```python
from build123d import *

# Parameters (mm, degrees)
F0_W        = 127
F0_H        = 88.9
F1_DEPTH    = 12.7
F2_T1_DEPTH = 177
F3_W        = 1.8
F3_H        = 6.85
F4_DEPTH    = 16.4
F3_W_2      = 7
F3_H_2      = 13.5
F3_W_3      = 2.7532497272
F3_H_3      = 12.2928316705
F5_DEPTH    = 16.4
F6_SIZE     = 1
F7_DEPTH    = 2.794
F8_DEPTH    = 1.8542
F3_R        = 3.9463270772
F9_DEPTH    = 0.762
F10_R       = 0.254
F13_W       = 127
F13_H       = 12.192
F14_DEPTH   = 0.5
F15_R       = 3.9211509086
F16_DEPTH   = 1.27


# Not quite as in the source:
# - a fillet or chamfer that OpenCascade refuses, or shapes differently, is made with other operations: its cross-section is extruded or revolved along the edge and cut away or added
# - the program builds the solid bodies; features that only make, move or delete a surface that nothing else refers to are left out


with BuildPart() as f1:
    # F0 (on Front) → F1 (new body)
    with BuildSketch(Plane.XZ):
        Rectangle(F0_W, F0_H)
    extrude(amount=F1_DEPTH)

    # F2: fillet of radius 10 on 4 edges, made by hand

    # F2_s2 → F2_t1 (cut)
    with BuildSketch(Plane.YZ.offset(-88.5)):
        with BuildLine():
            ThreePointArc((-2.7, 44.45), (-9.7710678119, 41.5210678119), (-12.7, 34.45))
            Line((-12.7, 34.45), (-12.7, 44.45))
            Line((-12.7, 44.45), (-2.7, 44.45))
        make_face()
        with BuildLine():
            ThreePointArc((-10, 44.45), (-2.9289321881, 41.5210678119), (0, 34.45))
            Line((0, 34.45), (0, 44.45))
            Line((0, 44.45), (-10, 44.45))
        make_face()
        with BuildLine():
            ThreePointArc((-2.7, -44.45), (-9.7710678119, -41.5210678119), (-12.7, -34.45))
            Line((-12.7, -34.45), (-12.7, -44.45))
            Line((-12.7, -44.45), (-2.7, -44.45))
        make_face()
        with BuildLine():
            ThreePointArc((-10, -44.45), (-2.9289321881, -41.5210678119), (0, -34.45))
            Line((0, -34.45), (0, -44.45))
            Line((0, -44.45), (-10, -44.45))
        make_face()
    extrude(amount=F2_T1_DEPTH, mode=Mode.SUBTRACT)

    # F3 (on face) → F4 (cut)
    with BuildSketch(Plane.YZ.offset(63.5)):
        with Locations((-7.1068273082, -6.4043554038)):
            Rectangle(F3_W, F3_H)
    extrude(amount=-F4_DEPTH, mode=Mode.SUBTRACT)

    # F3 (on face) → F5 (cut)
    with BuildSketch(Plane.YZ.offset(63.5)):
        with Locations((-6.591425851, 10.4809925538)):
            Rectangle(F3_W_2, F3_H_2)
        with Locations((-7.9680507146, 10.4750713799)):
            Rectangle(F3_W_3, F3_H_3, mode=Mode.SUBTRACT)
        with Locations((-6.591425851, 28.0195952505)):
            Rectangle(F3_W_2, F3_H_2)
        with Locations((-7.9680507146, 28.0764119234)):
            Rectangle(F3_W_3, F3_H_3, mode=Mode.SUBTRACT)
    extrude(amount=-F5_DEPTH, mode=Mode.SUBTRACT)

    # F6
    f6_edges = [f1.edges().sort_by_distance(p)[0] for p in [
        (55.3, -6.206827, -2.979355),
        (55.3, -6.206827, -9.829355),
    ]]
    chamfer(f6_edges, length=F6_SIZE)

    # F7 (add): faces of the model
    f7_faces = [f1.faces().sort_by_distance(p)[0] for p in [
        (63.5, -7.9680507146, 10.4750713799),
        (63.5, -7.9680507146, 28.0764119234),
    ]]
    extrude(f7_faces, amount=-F7_DEPTH)

    # F8 (cut): faces of the model
    f8_faces = [f1.faces().sort_by_distance(p)[0] for p in [
        (63.5, -7.9680507146, 10.4750713799),
        (63.5, -7.9680507146, 28.0764119234),
    ]]
    extrude(f8_faces, amount=-F8_DEPTH, mode=Mode.SUBTRACT)

    # F3 (on face) → F9 (join)
    with BuildSketch(Plane.YZ.offset(63.5)):
        with Locations((-6.3012135215, -31.0900993645)):
            Circle(F3_R)
    extrude(amount=F9_DEPTH)

    # F10
    f10_edges = [f1.edges().sort_by_distance(p)[0] for p in [
        (64.262, -10.247541, -31.090099),
    ]]
    fillet(f10_edges, radius=F10_R)

    # F13 (on face) → F14 (join)
    with BuildSketch(Plane.XZ.offset(12.7)):
        with Locations((0, 27.0355174699)):
            Rectangle(F13_W, F13_H)
        with Locations((-2.0266e-06, 13.3711864791)):
            Rectangle(F13_W, F13_H)
        with Locations((-2.0266e-06, -0.2175037199)):
            Rectangle(F13_W, F13_H)
        with Locations((-2.0266e-06, -13.8689222195)):
            Rectangle(F13_W, F13_H)
        with Locations((-2.0266e-06, -27.337996141)):
            Rectangle(F13_W, F13_H)
    extrude(amount=F14_DEPTH)

    # F15 (on face) → F16 (cut)
    with BuildSketch(Plane(origin=(-63.5, 0, 0), x_dir=(0, -1, 0), z_dir=(-1, 0, 0))):
        with Locations((7.0751463063, -30.106594786)):
            Circle(F15_R)
        with Locations((7.0751463063, 29.6837498702)):
            Circle(F15_R)
    extrude(amount=-F16_DEPTH, mode=Mode.SUBTRACT)

    # F17: fillet of radius 2.54 on 2 edges, made by hand

    # F17_s1 → F17_t2 (revolve)
    with BuildSketch(Plane.XY.offset(-30.106594786)):
        with BuildLine():
            ThreePointArc((-63.5, -10.9962972149), (-62.5702954744, -10.0665926893), (-62.23, -8.7965926893))
            Line((-62.23, -8.7965926893), (-62.23, -10.9962972149))
            Line((-62.23, -10.9962972149), (-63.5, -10.9962972149))
        make_face()
    revolve(axis=Axis((-62.23, -7.0751463063, -30.106594786), (-1, 0, 0)))

    # F17_s3 → F17_t4 (revolve)
    with BuildSketch(Plane.XY.offset(29.6837498702)):
        with BuildLine():
            ThreePointArc((-63.5, -10.9962972149), (-62.5702954744, -10.0665926893), (-62.23, -8.7965926893))
            Line((-62.23, -8.7965926893), (-62.23, -10.9962972149))
            Line((-62.23, -10.9962972149), (-63.5, -10.9962972149))
        make_face()
    revolve(axis=Axis((-62.23, -7.0751463063, 29.6837498702), (-1, 0, 0)))


solid = f1.part
```
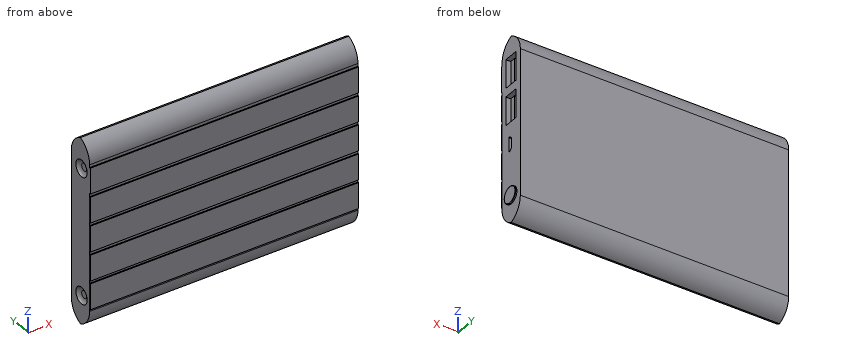
Here's how the part is built. I have some questions about the finished solid (model axes, mm). Round coordinates to 2 decimals unless told otherwise and drop trailing zeros. Order: outer loops, then holes, each group sorted by start corner. A loop starts at its lowest first (then second) coordinate and runs counter-clockwise, first axis right, second up. Notation, with made-up numbers: M 13,-37.75 L 51,-37.75 A21 cw 51,-30.75 Z; hole C 80.5,55.5 d9. An arc over 180 degrees is marked long. Answer in a Markdown table with one row per item.
Item 1: I'm going to push flat-ended pins straight in: pin 1 (7.5 mm diameter, centred on x = 59, y = -6, fed in from +Z); pin 2 (4 mm diameter, centred on y = -4.5, z = -14, fed in from +X); pin 3 (0.5 mm diameter, centred on y = -7.5, z = -7.5, fed in from +X); pin 4 (1.5 mm diameter, centred on x = -33, y = -5, fed in from -Z). Where does each tip first touch, or does it pass through?
A:
| item | result |
|---|---|
| pin 1 | stops at z = 43.76 |
| pin 2 | stops at x = 63.5 |
| pin 3 | stops at x = 47.1 |
| pin 4 | stops at z = -43.5 |
Item 2: If I drill on L1, parallel to Z at x = 51.5, y = -4.25; L2, parallel to X at y = -1, z = -4; L3, parallel to X at y = -8.5, z = 24, over which ranges is the centre line in solid material (lowest first)? Write a range as from..to.
A:
| item | result |
|---|---|
| L1 | z = -42.63..3.73, 17.23..21.27, 34.77..42.63 |
| L2 | x = -63.5..63.5 |
| L3 | x = -63.5..61.65 |
Item 3: Imagine slicing it at C-C, the plane z = -37. Write out the boundary of the cut face in (x, y), and give its area (3 significant figures).
A:
| item | result |
|---|---|
| outline | M -63.5,-12.37 L 63.5,-12.37 L 63.5,-0.33 L -63.5,-0.33 Z |
| area | 1,530 mm2 |
Item 4: Imagine slicing it at D-D, the plane z = 37.5. Write out the boundary of the cut face in (x, y).
A:
| item | result |
|---|---|
| outline | M -63.5,-12.22 L 63.5,-12.22 L 63.5,-0.48 L -63.5,-0.48 Z |
Item 5: Imagine slicing it at A-A, the plane z = 24.5. Write out the boundary of the cut face in (x, y), and give its area (3 significant figures).
A:
| item | result |
|---|---|
| outline | M -63.5,-13.2 L 63.5,-13.2 L 63.5,-10.09 L 47.1,-10.09 L 47.1,-9.34 L 61.65,-9.34 L 61.65,-6.59 L 47.1,-6.59 L 47.1,-3.09 L 63.5,-3.09 L 63.5,0 L -63.5,0 Z |
| area | 1,600 mm2 |
Item 6: Imagine slicing it at B-B, the plane x = -21.5. Write out the boundary of the cut face in (y, z).
A:
| item | result |
|---|---|
| outline | M -13.2,-33.43 L -12.7,-33.43 L -12.7,-34.45 A10 ccw -6.35,-43.76 A10 ccw 0,-34.45 L 0,34.45 A10 ccw -6.35,43.76 A10 ccw -12.7,34.45 L -12.7,33.13 L -13.2,33.13 L -13.2,20.94 L -12.7,20.94 L -12.7,19.47 L -13.2,19.47 L -13.2,7.28 L -12.7,7.28 L -12.7,5.88 L -13.2,5.88 L -13.2,-6.31 L -12.7,-6.31 L -12.7,-7.77 L -13.2,-7.77 L -13.2,-19.96 L -12.7,-19.96 L -12.7,-21.24 L -13.2,-21.24 Z |
